Verification items for this drawing (mm, ordinates from the low corner). Coordinates: 2 decimals unless noted, no trailing zeros. Loops run counter-clockwise (first coordinate to the right, second up) from the corner with the lowest first, then second, coordinate; pieces in that order, holes last. Notation, with made-up numbers: (80.25, 1) - (103.25, 1) arc R23 cw to (103.25, 40) - close; hole circle Ø9 at (42.5, 37). An arc over 180 degrees is marked (long way). One line per item, written item: value. Start each with the question number.
(1) Draft check along Z on the marked faces 1, 2 and 3. Enter one of: +Z half, -Z half, draft (parallel to the pull), parting line (faces both ways), or undercut.
(2) Section check A-A (x = 32.5). Record the boundary of the cut face in (y, z) (1 decimal).
(3) Section check C-C (x = 20). Record the boundary of the cut face in (y, z).
(4) Section check D-D (z = 59). Record the boundary of the cut face in (x, y).
(5) Gauge pin test, flat ends, axial feed: P1, Ø2.5, axis at x = 75, y = 10, coming from the -Z side; P2, Ø1, axis at y = 14.5, z = 47.5, coming from the -X side (1 decimal); P3, Ø6, axis at y = 2.5, z = 11, coming from the +X side (1 decimal). Record the tip position at first contact, or that the pin passes through.
(6) Section check B-B (x = 75). Record the boundary of the cut face in (y, z) (1 decimal).
(7) Thickness scan on probe 1 along Y at (x, z) = (75, 47.4) (1 decimal); probe 2 along Z at (x, y) = (69, 10); probe 3 along Y at (x, z) = (78, 43). Record the ranges inside material, lowest first. Write a range as [from, to].
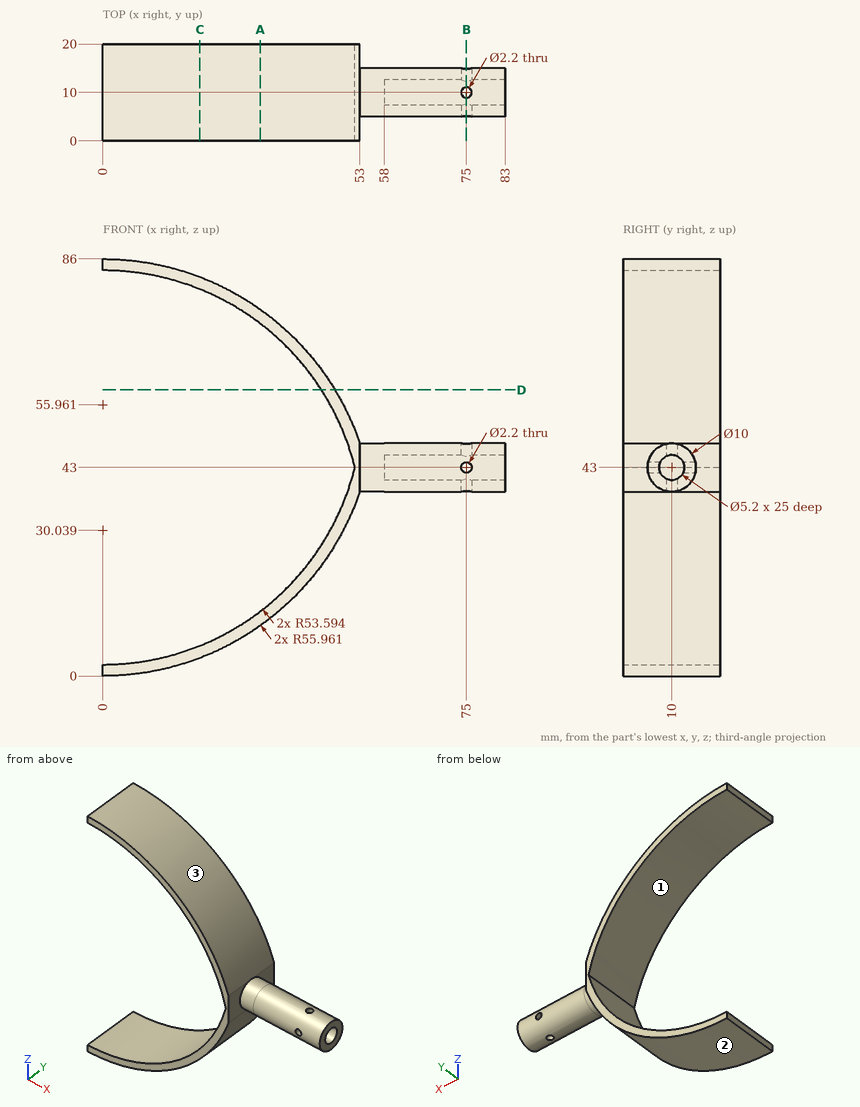
Responses:
1. face 1: undercut
1. face 2: -Z half
1. face 3: +Z half
2. outline: (0, 10.4) - (20, 10.4) - (20, 13.3) - (0, 13.3) - close; (0, 72.7) - (20, 72.7) - (20, 75.6) - (0, 75.6) - close
3. outline: (0, 3.7) - (20, 3.7) - (20, 6.24) - (0, 6.24) - close; (0, 79.76) - (20, 79.76) - (20, 82.3) - (0, 82.3) - close
4. outline: (45.1, 0) - (47.88, 0) - (47.88, 20) - (45.1, 20) - close
5. P1: stops at z = 38
5. P2: stops at x = 50.5
5. P3: stops at x = 37
6. outline: (5.1, 41.9) arc R5 ccw to (8.9, 38.1) - (8.9, 40.6) arc R2.6 cw to (7.6, 41.9) - close; (5.1, 44.1) - (7.6, 44.1) arc R2.6 cw to (8.9, 45.4) - (8.9, 47.9) arc R5 ccw to start; (11.1, 38.1) arc R5 ccw to (14.9, 41.9) - (12.4, 41.9) arc R2.6 cw to (11.1, 40.6) - close; (11.1, 45.4) arc R2.6 cw to (12.4, 44.1) - (14.9, 44.1) arc R5 ccw to (11.1, 47.9) - close
7. probe 1: y = [7.6, 8.9], [11.1, 12.4]
7. probe 2: z = [38, 40.4], [45.6, 48]
7. probe 3: y = [5, 7.4], [12.6, 15]
